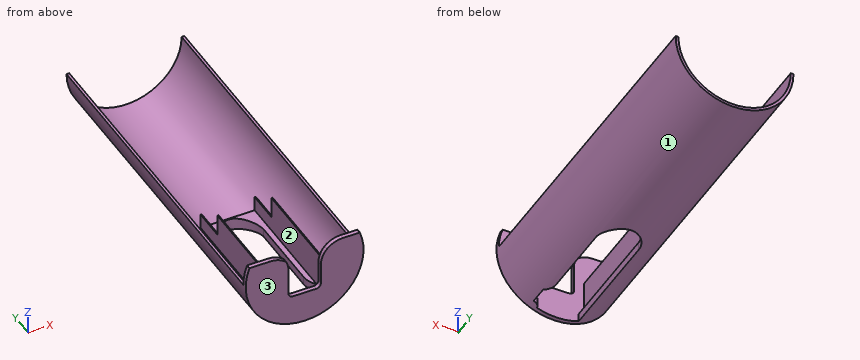
from build123d import *

# Parameters (mm, degrees)
SKETCH1_R               = 25.7
MAIN_CYLINDER_DEPTH     = 150
SKETCH4_R               = 24.5
MAIN_CUT_DOWN_DEPTH     = 148
SKETCH7_W               = 24.1
SKETCH7_H               = 31
FEATHER_BOX_DEPTH       = 62
FEATHER_HOLE_DEPTH      = 90
FEATHER_HOLE_DEPTH_BACK = 62
SKETCH8_W               = 23.1
SKETCH8_H               = 32
WINDOW_START            = 62
WINDOW_FILLER_DEPTH     = 62
SKETCH18_W              = 18.3
SKETCH18_H              = 50
WINDOW_CUT_DEPTH        = 16
SD_RESET_ACCESS_DEPTH   = 2
SKETCH26_W              = 0.5
SKETCH26_H              = 62
TRIM_DEPTH              = 15
FILLET3_R               = 10
SKETCH34_W              = 49.114786026
SKETCH34_H              = 17.457477886
CUT_EXTRUDE5_DEPTH      = 2
FILLET7_R               = 10
FILLET8_R               = 10
FILLET9_R               = 2
SKETCH28_W              = 2.4
SKETCH28_H              = 8
CUT_EXTRUDE6_DEPTH      = 10
FILLET10_R              = 10
FILLET11_R              = 2
SKETCH35_W              = 0.5
SKETCH35_H              = 9.444605522
CUT_EXTRUDE7_DEPTH      = 14


# Some blends are built 0.0001 mm under size
with BuildPart() as part:
    # Sketch1 → Main Cylinder (new body)
    with BuildSketch(Plane(origin=(0, 0, 0), x_dir=(1, 0, 0), z_dir=(0, 1, 0))):
        with Locations(Location((0, 0, 0), (0, 0, 270))):
            Circle(SKETCH1_R)
    extrude(amount=MAIN_CYLINDER_DEPTH)

    # Sketch4 → Main cut down (cut)
    with BuildSketch(Plane(origin=(0, 150, 0), x_dir=(1, 0, 0), z_dir=(0, 1, 0))):
        Circle(SKETCH4_R)
        Polygon((0, 0), (25.7, 0), (25.7, -40.6), (-25.7, -40.6), (-25.7, 0), align=None)
    extrude(amount=-MAIN_CUT_DOWN_DEPTH, mode=Mode.SUBTRACT)

    # Sketch7 → Feather box (add)
    with BuildSketch(Plane(origin=(0, 2, 0), x_dir=(1, 0, 0), z_dir=(0, 1, 0))):
        with Locations((0, 4.951216806)):
            Rectangle(SKETCH7_W, SKETCH7_H)
    extrude(amount=FEATHER_BOX_DEPTH)

    # Sketch8 → Feather hole (cut, two sides: drawn at the far end of the back side and taken through both)
    with BuildSketch(Plane(origin=(0, 64, 0), x_dir=(1, 0, 0), z_dir=(0, 1, 0)).offset(-FEATHER_HOLE_DEPTH_BACK)):
        with Locations((0, 4.451216806)):
            Rectangle(SKETCH8_W, SKETCH8_H)
    extrude(amount=FEATHER_HOLE_DEPTH + FEATHER_HOLE_DEPTH_BACK, mode=Mode.SUBTRACT)

    # Sketch15 → window filler (add)
    with BuildSketch(Plane(origin=(0, 2, 0), x_dir=(1, 0, 0), z_dir=(0, 1, 0)).offset(WINDOW_START)):
        with BuildLine():
            Line((-13.575571615, 20.394946809), (13.575571615, 20.394946809))
            ThreePointArc((13.575571615, 20.394946809), (0, 24.5), (-13.575571615, 20.394946809))
        make_face()
    extrude(amount=-WINDOW_FILLER_DEPTH)

    # Sketch18 → window cut (cut)
    with BuildSketch(Plane.XY.offset(-20.394946809)):
        with BuildLine():
            add(Edge.make_bspline(
                [(-9.15, 52), (-9.166701282, 56.998161016), (-0.16215998, 69.276496907), (8.559054188, 57.202948769), (9.892970994, 47.089830129), (-8.678000401, 46.988029764), (-9.148278475, 51.484802374), (-9.15, 52)],
                knots=[0, 0, 0, 0, 0.329948679, 0.626902491, 0.693907623, 0.965989736, 1, 1, 1, 1], degree=3))
        make_face()
        with Locations((0, 27)):
            Rectangle(SKETCH18_W, SKETCH18_H)
    extrude(amount=-WINDOW_CUT_DEPTH, mode=Mode.SUBTRACT)

    # Sketch23 → sd reset access (cut)
    with BuildSketch(Plane(origin=(0, 2, 0), x_dir=(1, 0, 0), z_dir=(0, 1, 0))):
        Polygon((-8.05, -11.21), (9.8, -11.21), (9.8, -6.21), (7.05, -6.21), (7.05, 11.79), (-7.05, 11.79), (-7.05, -6.21), (-8.05, -6.21), align=None)
    extrude(amount=-SD_RESET_ACCESS_DEPTH, mode=Mode.SUBTRACT)

    # Sketch26 → trim (cut)
    with BuildSketch(Plane.XY.offset(10.548783194)):
        with Locations((-11.8, 33)):
            Rectangle(SKETCH26_W, SKETCH26_H)
        with Locations((11.8, 33)):
            Rectangle(SKETCH26_W, SKETCH26_H)
    extrude(amount=-TRIM_DEPTH, mode=Mode.SUBTRACT)

    # Fillet3
    # the kernel refuses this fillet: 10 mm, written as the material it takes off along each edge
    with BuildSketch(Plane(origin=(-7.05, 12.897247359, 6.21), x_dir=(0, 0, -1), z_dir=(0, -1, 0))) as fillet3_piece_1:
        with BuildLine():
            CenterArc((4.358898944, -10), FILLET3_R, 90, 25.841932763)
            Line((0, -1), (-0.087177979, -0.82))
            ThreePointArc((-0.087177979, -0.82), (-0.2, -0.5), (-0.2, 0))
            Line((-0.2, 0), (0, 0.2))
            Line((0, 0.2), (4.358898944, 0.2))
            Line((4.358898944, 0.2), (4.358898944, 0))
        make_face()
    extrude(amount=23.794494718, mode=Mode.SUBTRACT)

    # Sketch34 → Cut-Extrude5 (cut)
    with BuildSketch(Plane(origin=(0, 2, 0), x_dir=(1, 0, 0), z_dir=(0, 1, 0))):
        with Locations((-0.549154382, -17.755029201)):
            Rectangle(SKETCH34_W, SKETCH34_H)
    extrude(amount=-CUT_EXTRUDE5_DEPTH, mode=Mode.SUBTRACT)

    # Fillet7
    # the kernel refuses this fillet: 10 mm, written as the material it takes off along each edge
    with BuildSketch(Plane(origin=(-8.05, 19.391505532, 9.026290258), x_dir=(-1, 0, 0), z_dir=(0, -1, 0))) as fillet7_piece_1:
        with BuildLine():
            CenterArc((6.956602213, 10), FILLET7_R, 225.920148316, 44.079851684)
            Line((0, 2.816290258), (-0.139132044, 2.672616063))
            ThreePointArc((-0.139132044, 2.672616063), (-0.2, 1.408145129), (-0.2, 0))
            Line((-0.2, 0), (0, -0.2))
            Line((0, -0.2), (6.956602213, -0.2))
            Line((6.956602213, -0.2), (6.956602213, 0))
        make_face()
    extrude(amount=36.783011063, mode=Mode.SUBTRACT)

    # Fillet8
    # the kernel refuses this fillet: 10 mm, written as the material it takes off along each edge
    with BuildSketch(Plane(origin=(9.8, -17.391505532, 9.026290258), x_dir=(1, 0, 0), z_dir=(0, 1, 0))) as fillet8_piece_1:
        with BuildLine():
            CenterArc((6.956602213, 10), FILLET8_R, 225.920148316, 44.079851684)
            Line((0, 2.816290258), (-0.139132044, 2.672616063))
            ThreePointArc((-0.139132044, 2.672616063), (-0.2, 1.408145129), (-0.2, 0))
            Line((-0.2, 0), (0, -0.2))
            Line((0, -0.2), (6.956602213, -0.2))
            Line((6.956602213, -0.2), (6.956602213, 0))
        make_face()
    extrude(amount=36.783011063, mode=Mode.SUBTRACT)
    with BuildSketch(Plane(origin=(7.05, 19.218721642, 6.21), x_dir=(1, 0, 0), z_dir=(0, -1, 0))) as fillet8_piece_2:
        with BuildLine():
            CenterArc((10, -6.887488657), FILLET8_R, 136.468847833, 43.531152167)
            Line((0, -6.887488657), (-0.2, -6.887488657))
            Line((-0.2, -6.887488657), (-0.2, 0))
            Line((-0.2, 0), (0, 0.2))
            ThreePointArc((0, 0.2), (1.375, 0.2), (2.605, 0.137749773))
            Line((2.605, 0.137749773), (2.75, 0))
        make_face()
    extrude(amount=36.437443285, mode=Mode.SUBTRACT)

    # Fillet9
    fillet9_edges = [part.edges().sort_by_distance(p)[0] for p in [
        (-7.05, 1, -11.79),
        (7.05, 1, -11.79),
    ]]
    fillet(fillet9_edges, radius=FILLET9_R)

    # Sketch28 → Cut-Extrude6 (cut)
    with BuildSketch(Plane.XY.offset(-20.394946809)):
        with Locations((10.35, 8)):
            Rectangle(SKETCH28_W, SKETCH28_H)
    extrude(amount=-CUT_EXTRUDE6_DEPTH, mode=Mode.SUBTRACT)

    # Fillet10
    # the kernel refuses this fillet: 10 mm, written as the material it takes off along each edge
    with BuildSketch(Plane(origin=(9.15, 12, -4.146869999), x_dir=(1, 0, 0), z_dir=(0, 0, -1))) as fillet10_piece_1:
        with BuildLine():
            CenterArc((10, -6.499230724), FILLET10_R, 139.464197889, 40.535802111)
            Line((0, -6.499230724), (-0.2, -6.499230724))
            Line((-0.2, -6.499230724), (-0.2, 0))
            Line((-0.2, 0), (0, 0.2))
            ThreePointArc((0, 0.2), (1.2, 0.2), (2.248, 0.129984614))
            Line((2.248, 0.129984614), (2.4, 0))
        make_face()
    extrude(amount=36.117191071, mode=Mode.SUBTRACT)

    # Fillet11
    fillet11_edges = [part.edges().sort_by_distance(p)[0] for p in [
        (9.15, 4, -22.205465534),
    ]]
    fillet(fillet11_edges, radius=FILLET11_R - 0.0001)  # a hair under: the kernel refuses the full size

    # Sketch35 → Cut-Extrude7 (cut)
    with BuildSketch(Plane(origin=(0, 64, 0), x_dir=(1, 0, 0), z_dir=(0, 1, 0))):
        with Locations((-11.8, 9.173519567)):
            Rectangle(SKETCH35_W, SKETCH35_H)
        with Locations((11.8, 9.173519567)):
            Rectangle(SKETCH35_W, SKETCH35_H)
    extrude(amount=-CUT_EXTRUDE7_DEPTH, mode=Mode.SUBTRACT)


solid = part.part
Read the model definition and answer for the solid it produces. Units are mm, in the model's axes. Face numbers are marked on the shaded views. Coordinates: 2 decimals unless noted, no trailing zeros. Order: outer loops, then holes, each group sorted by start corner. A loop starts at its lowest first (then second) coordinate and runs counter-clockwise, first axis right, second up. Notation, with made-up numbers: (-3, 33) -> (5, 33) arc R23 ccw to (5, 59) -> close; hole circle Ø5 at (16, -36). An arc over 180 degrees is marked (long way). Answer as a JSON object with one key per item and string values.
1) A cutting plane is placed at B-B, the plane y = 31. Determine the outline of the cut face in (x, z).
Model answer:
{"outline": "(-25.7, 0) arc R25.7 ccw to (-9.15, -24.02) -> (-9.15, -20.39) -> (-11.55, -20.39) -> (-11.55, -4.45) -> (-12.05, -4.45) -> (-12.05, -20.39) -> (-13.58, -20.39) arc R24.5 cw to (-24.5, 0) -> close; (9.15, -24.02) arc R25.7 ccw to (25.7, 0) -> (24.5, 0) arc R24.5 cw to (13.58, -20.39) -> (12.05, -20.39) -> (12.05, -4.45) -> (11.55, -4.45) -> (11.55, -20.39) -> (9.15, -20.39) -> close"}
2) Consider line 1 along X through (y, z) = (38, -11.5); line 2 along X through (y, z) = (13, -10); line 3 along Y through (x, z) = (5.5, -18). Determine where each line is inside the solid, lowest interval first. Write a range as from..to.
Model answer:
{"line 1": "x = -22.98..-21.63, -12.05..-11.55, 11.55..12.05, 21.63..22.98", "line 2": "x = -23.67..-22.37, -12.05..-11.55, 11.55..12.05, 22.37..23.67", "line 3": "y = 0..2"}
3) The mould has two halves that part along X. Classify the marked faces 1, 2 and 3: released by +X, released by -X, zero draft, split by the parting line, or undercut.
Model answer:
{"face 1": "split by the parting line", "face 2": "undercut", "face 3": "zero draft"}
4) A cutting plane is placed at C-C, the plane x = -19. Determine the outline of the cut face in (y, z), plus the area to 3 significant figures.
Model answer:
{"outline": "(0, -17.31) -> (150, -17.31) -> (150, -15.47) -> (2, -15.47) -> (2, 9.03) -> (0, 9.03) -> close", "area": "325 mm²"}
5) A cutting plane is placed at A-A, the plane y = 10. Determine the outline of the cut face in (x, z), plus the area to 3 significant figures.
Model answer:
{"outline": "(-25.7, 0) arc R25.7 ccw to (-9.15, -24.02) -> (-9.15, -20.39) -> (-11.55, -20.39) -> (-11.55, -4.45) -> (-12.05, -4.45) -> (-12.05, -20.39) -> (-13.58, -20.39) arc R24.5 cw to (-24.5, 0) -> close; (11.55, -22.96) arc R25.7 ccw to (25.7, 0) -> (24.5, 0) arc R24.5 cw to (13.58, -20.39) -> (12.05, -20.39) -> (12.05, -4.45) -> (11.55, -4.45) -> close", "area": "91.8 mm²"}
6) Each of these flat-tipped pins is pushed along its axis until it touches: pin 1 (1.6 mm diameter, centred on x = 10, y = 3.5, fed in from +Z); pin 2 (1 mm diameter, centred on x = -0.5, y = 1.5, fed in from +Z); pin 3 (0.6 mm diameter, centred on x = 12, z = -10, fed in from +Y). Where does it stop, or does it pass through?
Model answer:
{"pin 1": "stops at z = -20.39", "pin 2": "stops at z = -11.79", "pin 3": "stops at y = 50"}
7) A cutting plane is placed at D-D, the plane y = 125. Determine the outline of the cut face in (x, z), plus the area to 3 significant figures.
Model answer:
{"outline": "(-25.7, 0) arc R25.7 ccw to (25.7, 0) -> (24.5, 0) arc R24.5 cw to (-24.5, 0) -> close", "area": "94.6 mm²"}
